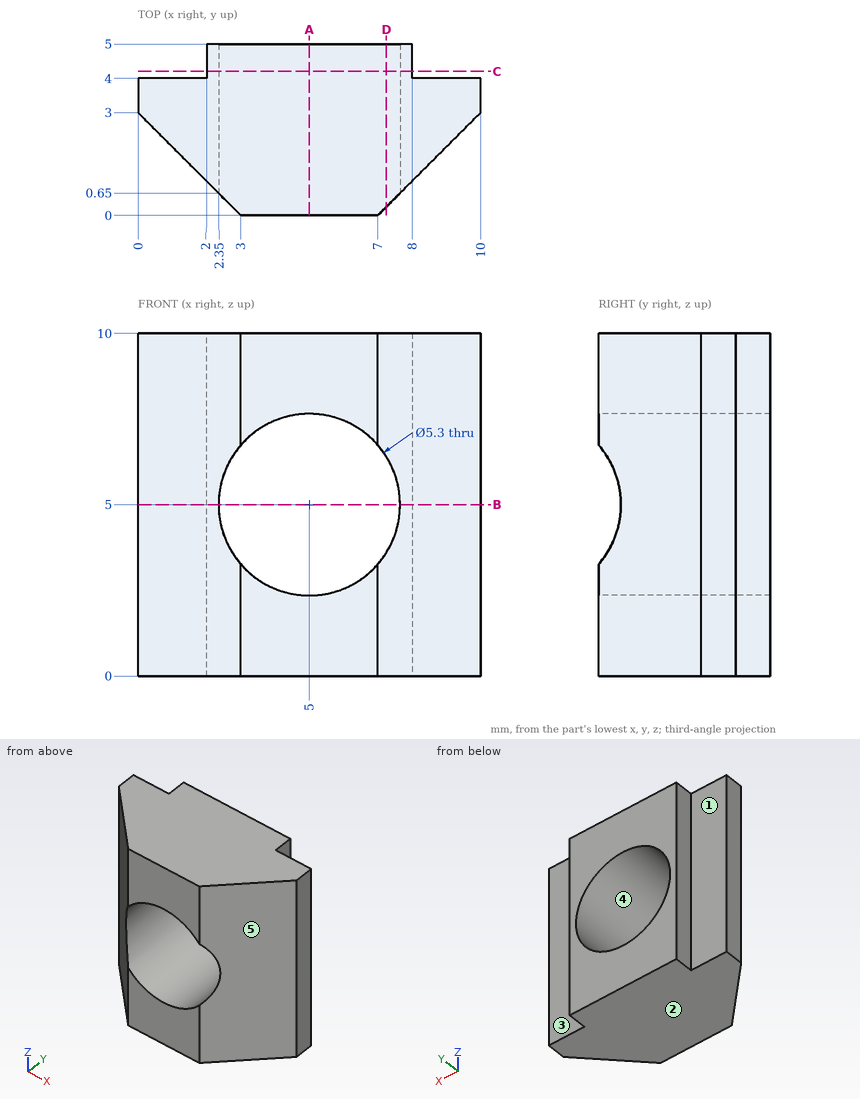
The figure shows three views and two pictorial views of one solid part (mm, origin at its lowest corner). Answer the questions. A direction names the side the tool comes from. Give positions to 0.01 mm unless a question says otherwise; leave off trailing zeros. Write each loop counter-clockwise with the first axis right and the second up, starting at its lowest first coordinate (ties: lowest second). Pieces come first, ordered by that corner, then holes. Notation, with made-up numbers: M 47,1.5 L 79,1.5 A12 ccw 79,5.5 Z; hole C 34,22 d4. An arc over 180 degrees is marked long. One line per item, written item: value. Start each with the question number.
(1) Find section B-B (z = 5). Determine the outline of the cut face in (x, y), plus the area to 3 significant figures.
(2) Find section A-A (x = 5). Determine the outline of the cut face in (y, z), plus the area to 3 significant figures.
(3) Find section D-D (x = 7.25). Determine the outline of the cut face in (y, z).
(4) Determine the mould class of the marked faces 3, 4 and 5 for opening direction X: pulls with the +X half, pulls with the -X half, needs draft (parallel to the pull), parting line crosses it, or undercut.
(5) Find the intervals of material crossed by line 1 (Z direction, x = 5, y = 1.8); line 2 (X direction, y = 4.25, z = 8.25); line 3 (Y direction, x = 1, z = 7.75), in increasing order.
(6) A tool of negligible diameter and unlimited length cuts with its end or side. For the marked faces 1 and 2, from which of +Z, -Z, +X, -X, +Y, -Y can it reach the whole face along a straight path? Write none if from no direction.
(7) Find section C-C (y = 4.2). Determine the outline of the cut face in (x, z).
(8) Flat-ended cylindrical pins translate along their axes: pin 1 Ø1.5 at (x, z) = (8, 7.5) entering from -Y; pin 2 Ø3 at (x, z) = (4, 5) entering from -Y; pin 3 Ø0.6 at (x, z) = (8.5, 4) entering from +Y. Find the tip coordinate at first contact, or state that the pin passes through.
Results below:
1. outline: M 0,3 L 2.35,0.65 L 2.35,5 L 2,5 L 2,4 L 0,4 Z; M 7.65,0.65 L 10,3 L 10,4 L 8,4 L 8,5 L 7.65,5 Z
1. area: 10.9 mm^2
2. outline: M 0,0 L 5,0 L 5,2.35 L 0,2.35 Z; M 0,7.65 L 5,7.65 L 5,10 L 0,10 Z
2. area: 23.5 mm^2
3. outline: M 0.25,0 L 5,0 L 5,3.6 L 0.25,3.6 Z; M 0.25,6.4 L 5,6.4 L 5,10 L 0.25,10 Z
4. face 3: needs draft
4. face 4: undercut
4. face 5: pulls with the +X half
5. line 1: z = 0 to 2.35, 7.65 to 10
5. line 2: x = 2 to 8
5. line 3: y = 2 to 4
6. face 1: +Z, -Z, -X, +Y
6. face 2: -Z, +X, -X, +Y, -Y
7. outline: M 2,0 L 8,0 L 8,10 L 2,10 Z; hole C 5,5 d5.3
8. pin 1: stops at y = 0.25
8. pin 2: passes through
8. pin 3: stops at y = 4
